```python
from build123d import *

# Parameters (mm, degrees)
SKETCH1_W            = 26.5
SKETCH1_H            = 5.6
BOSS_EXTRUDE1_DEPTH  = 1.056
SKETCH2_W            = 10
SKETCH2_H            = 4.2
BOSS_EXTRUDE2_DEPTH  = 1.7
FILLET1_R            = 1.5
FILLET2_R            = 1.3
FILLET3_R            = 0.4
FILLET2_OF_MIRROR2_R = 1.3
FILLET3_OF_MIRROR2_R = 0.4


with BuildPart() as part:
    # Sketch1 → Boss-Extrude1 (new body)
    with BuildSketch(Plane(origin=(0, 0, 0), x_dir=(1, 0, 0), z_dir=(0, 1, 0))):
        Rectangle(SKETCH1_W, SKETCH1_H)
    extrude(amount=BOSS_EXTRUDE1_DEPTH)

    # Sketch2 → Boss-Extrude2 (add)
    with BuildSketch(Plane(origin=(0, 1.056, 0), x_dir=(1, 0, 0), z_dir=(0, 1, 0))):
        with Locations((7.465, 0)):
            Rectangle(SKETCH2_W, SKETCH2_H)
    boss_extrude2 = extrude(amount=BOSS_EXTRUDE2_DEPTH)

    # Fillet1
    fillet1_edges = [part.edges().sort_by_distance(p)[0] for p in [
        (13.25, 0.528, 2.8),
        (-13.25, 0.528, 2.8),
        (-13.25, 0.528, -2.8),
        (13.25, 0.528, -2.8),
    ]]
    fillet(fillet1_edges, radius=FILLET1_R)

    # Fillet2
    fillet2_edges = [part.edges().sort_by_distance(p)[0] for p in [
        (12.465, 1.906, 2.1),
        (12.465, 1.906, -2.1),
        (2.465, 1.906, -2.1),
        (2.465, 1.906, 2.1),
    ]]
    fillet(fillet2_edges, radius=FILLET2_R)

    # Fillet3
    fillet3_edges = [part.edges().sort_by_distance(p)[0] for p in [
        (2.465, 2.756, 0),
        (7.465, 2.756, -2.1),
        (12.465, 2.756, 0),
        (7.465, 2.756, 2.1),
        (2.845761184, 2.756, 1.719238816),
        (12.084238816, 2.756, 1.719238816),
        (12.084238816, 2.756, -1.719238816),
        (2.845761184, 2.756, -1.719238816),
    ]]
    fillet(fillet3_edges, radius=FILLET3_R)

    # Mirror2: Boss-Extrude2 across plane
    add(boss_extrude2.mirror(Plane(origin=(0, 0, 0), x_dir=(0, 0, 1), z_dir=(1, 0, 0))))

    # Fillet2 of Mirror2
    fillet2_of_mirror2_edges = [part.edges().sort_by_distance(p)[0] for p in [
        (-12.465, 1.906, 2.1),
        (-12.465, 1.906, -2.1),
        (-2.465, 1.906, -2.1),
        (-2.465, 1.906, 2.1),
    ]]
    fillet(fillet2_of_mirror2_edges, radius=FILLET2_OF_MIRROR2_R)

    # Fillet3 of Mirror2
    fillet3_of_mirror2_edges = [part.edges().sort_by_distance(p)[0] for p in [
        (-2.465, 2.756, 0),
        (-7.465, 2.756, -2.1),
        (-12.465, 2.756, 0),
        (-7.465, 2.756, 2.1),
        (-2.845761184, 2.756, 1.719238816),
        (-12.084238816, 2.756, 1.719238816),
        (-12.084238816, 2.756, -1.719238816),
        (-2.845761184, 2.756, -1.719238816),
    ]]
    fillet(fillet3_of_mirror2_edges, radius=FILLET3_OF_MIRROR2_R)


solid = part.part
```
Can you work these out from the model? Positions are in its coordinate system, mm. A direction names the side the tool comes from. Give positions to 0.01 mm unless a question says otherwise; leave off trailing zeros. Order: outer loops, then holes, each group sorted by start corner. A loop starts at its lowest first (then second) coordinate and runs counter-clockwise, first axis right, second up. Notation, with made-up numbers: (56, -19) - (102, -19) arc R34 cw to (102, 17) - close; hole circle Ø6 at (-5, 33). An arc over 180 degrees is marked (long way). Use a Markdown table: item, result. Add a question column.
Q1. If we section it at B-B on x = 9.5: Write out the boundary of the cut face in (y, z).
Q2. I'm going to push flat-ended pins straight in: pin 1 (1 mm diameter, centred on y = 1.5, z = -0.5, fed in from +X); pin 2 (0.7 mm diameter, centred on x = -6, y = 2, fed in from +Z); pin 3 (1.4 mm diameter, centred on x = 8, y = 2, fed in from -Z); pin 4 (1 mm diameter, centred on y = 2, z = 0, fed in from -X) (3 decimals). Where does each tip first touch, or does it pass through?
Q3. If we section it at C-C on z = -0.25: Write out the boundary of the cut face in (x, y) (3 decimals), plus the area to 3 significant figures.
Q4. On a 3-axis mill with a long thin cutter (end or side, diameter ignored), from which of +Z, -Z, +X, -X, +Y, -Y can I reach the whole of each face in a straight line? I mean faces 1 (the cylindrical face through (2.856, 1.715, -1.729)), 2 (the cylindrical face through (2.856, 1.715, 1.729)), 3 (the flat face through (7, 2, 2.1)). Say none if no direction works.
Q5. Please list where these lines run through material, in increasing order: line 1 along X through (y, z) = (1.55, 0.75) (3 decimals); line 2 along Z through (x, y) = (-10.25, 1.65); line 3 along Y through (x, z) = (-1.25, -0.95).
Q6. If we section it at A-A on y = 1.3: Write out the boundary of the cut face in (x, z) (3 decimals).
Q7. If we section it at D-D on x = -1.25: Write out the boundary of the cut face in (y, z), plus the area to 3 significant figures.
Answers follow:
| question | item | result |
|---|---|---|
| 1 | outline | (0, -2.8) - (1.06, -2.8) - (1.06, -2.1) - (2.36, -2.1) arc R0.4 ccw to (2.76, -1.7) - (2.76, 1.7) arc R0.4 ccw to (2.36, 2.1) - (1.06, 2.1) - (1.06, 2.8) - (0, 2.8) - close |
| 2 | pin 1 | stops at x = 13.25 |
| 2 | pin 2 | stops at z = 2.1 |
| 2 | pin 3 | stops at z = -2.1 |
| 2 | pin 4 | stops at x = -12.465 |
| 3 | outline | (-13.25, 0) - (13.25, 0) - (13.25, 1.056) - (12.465, 1.056) - (12.465, 2.356) arc R0.4 ccw to (12.065, 2.756) - (2.865, 2.756) arc R0.4 ccw to (2.465, 2.356) - (2.465, 1.056) - (-2.465, 1.056) - (-2.465, 2.356) arc R0.4 ccw to (-2.865, 2.756) - (-12.065, 2.756) arc R0.4 ccw to (-12.465, 2.356) - (-12.465, 1.056) - (-13.25, 1.056) - close |
| 3 | area | 61.8 mm^2 |
| 4 | face 1 | -Z, +Y |
| 4 | face 2 | +Z, +Y |
| 4 | face 3 | +Z, +X, -X, +Y |
| 5 | line 1 | x = -12.465 to -2.465, 2.465 to 12.465 |
| 5 | line 2 | z = -2.1 to 2.1 |
| 5 | line 3 | y = 0 to 1.06 |
| 6 | outline | (-12.465, -0.8) arc R1.3 ccw to (-11.165, -2.1) - (-3.765, -2.1) arc R1.3 ccw to (-2.465, -0.8) - (-2.465, 0.8) arc R1.3 ccw to (-3.765, 2.1) - (-11.165, 2.1) arc R1.3 ccw to (-12.465, 0.8) - close; (2.465, -0.8) arc R1.3 ccw to (3.765, -2.1) - (11.165, -2.1) arc R1.3 ccw to (12.465, -0.8) - (12.465, 0.8) arc R1.3 ccw to (11.165, 2.1) - (3.765, 2.1) arc R1.3 ccw to (2.465, 0.8) - close |
| 7 | outline | (0, -2.8) - (1.06, -2.8) - (1.06, 2.8) - (0, 2.8) - close |
| 7 | area | 5.91 mm^2 |
